```python
from build123d import *

# Parameters (mm, degrees)
F0_W     = 550
F0_H     = 450
F1_DEPTH = 5
F2_T     = -2
F4_D     = 15


with BuildPart() as f1:
    # F0 (on Front) → F1 (new body)
    with BuildSketch(Plane.XZ):
        Rectangle(F0_W, F0_H)
    extrude(amount=F1_DEPTH)

    # F2
    f2_openings = [f1.faces().sort_by_distance(p)[0] for p in [
        (0, -5, 0),
    ]]
    offset(amount=F2_T, openings=f2_openings)

    # F4 (through all)
    with Locations(Plane(origin=(0, 0, 0), x_dir=(-1, 0, 0), z_dir=(0, 1, 0))):
        with Locations((235, 0), (-235, 0), (-200, -175), (200, -175)):
            Hole(F4_D / 2)


solid = f1.part
```
Model file for the job. Use its own axes, mm. A direction names the side the tool comes from. Round coordinates to 2 decimals unless told otherwise and drop trailing zeros. Order: outer loops, then holes, each group sorted by start corner. A loop starts at its lowest first (then second) coordinate and runs counter-clockwise, first axis right, second up. Notation, with made-up numbers: (85, -7) -> (125, -7) arc R17 ccw to (125, 24) -> close; hole circle Ø5 at (61, 14.25). An arc over 180 degrees is marked (long way). Use one line per item in the form item = value.
Item 1: Drill centre lines: line 1 (Z direction, x = 235, y = -0.6); line 2 (X direction, y = -3.35, z = -162.5); line 3 (Z direction, x = -200, y = -0.65). Where is each one in solid material? Low to high.
Returned:
line_1 = -225 to -7.5, 7.5 to 225
line_2 = -275 to -273, 273 to 275
line_3 = -225 to -182.5, -167.5 to 225
Item 2: Cut at C-C, the plane y = -3.7. Write the cut outline in (x, z), and give its area (3 significant figures).
Returned:
outline = (-275, -225) -> (275, -225) -> (275, 225) -> (-275, 225) -> close; hole (-273, -223) -> (273, -223) -> (273, 223) -> (-273, 223) -> close
area = 3,980 mm^2
Item 3: Cut at A-A, the plane z = -175. Write the cut outline in (x, y).
Returned:
outline = (-275, -5) -> (-273, -5) -> (-273, -2) -> (-207.5, -2) -> (-207.5, 0) -> (-275, 0) -> close; (-192.5, -2) -> (192.5, -2) -> (192.5, 0) -> (-192.5, 0) -> close; (207.5, -2) -> (273, -2) -> (273, -5) -> (275, -5) -> (275, 0) -> (207.5, 0) -> close
Item 4: Cut at D-D, the plane x = 104.5. Write the cut outline in (y, z).
Returned:
outline = (-5, -225) -> (0, -225) -> (0, 225) -> (-5, 225) -> (-5, 223) -> (-2, 223) -> (-2, -223) -> (-5, -223) -> close
Item 5: Cut at B-B, the plane x = 235. Write the cut outline in (y, z).
Returned:
outline = (-5, -225) -> (0, -225) -> (0, -7.5) -> (-2, -7.5) -> (-2, -223) -> (-5, -223) -> close; (-5, 223) -> (-2, 223) -> (-2, 7.5) -> (0, 7.5) -> (0, 225) -> (-5, 225) -> close
Item 6: Flat gauge pins, fed straight in: pin 1 Ø4 at (x, z) = (-10.5, 75) entering from +Y; pin 2 Ø13.5 at (x, z) = (-200, -175) entering from +Y; pin 3 Ø19.5 at (x, z) = (200, -175) entering from -Y. Where does each tip first touch, or does it go through?
Returned:
pin_1 = 0
pin_2 = through
pin_3 = -2
Item 7: Tool access for faces 1 (the face through (227.507, -1.014, 0.33)), 2 (the face through (-4, -2, 3)): list every direction of +Z, -Z, +X, -X, +Y, -Y with a clear straight run to the whole face (end or side of a thin tool).
Returned:
face_1 = +Y, -Y
face_2 = -Y
Item 8: Pull direction X, two halves, no side cores. Call faces 3 (the face through (-4, 0, 3)), 4 (the face through (-242.493, -1.014, 0.33)): released by +X, released by -X, zero draft, split by the parting line, or undercut.
Returned:
face_3 = zero draft
face_4 = undercut
